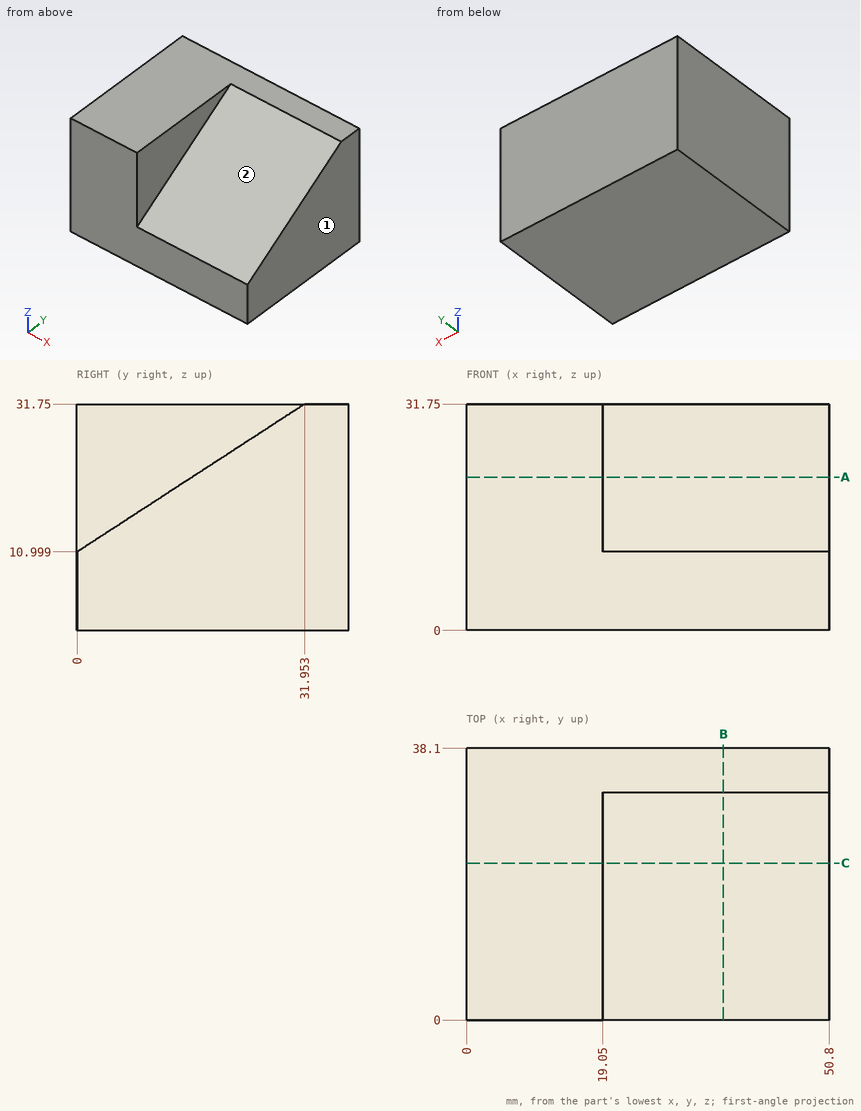
Here's the drawing with two shaded views (mm, measured from the low corner). I have some questions. A direction names the side the tool comes from. Give positions to 0.01 mm unless a question says otherwise; leave off trailing zeros. Loops run counter-clockwise (first coordinate to the right, second up) from the corner with the lowest first, then second, coordinate; pieces in that order, holes last. Notation, with made-up numbers: (64.25, -0.5) - (103.25, -0.5) arc R13 cw to (103.25, 8.5) - close; hole circle Ø2 at (-36, 86.25). An arc over 180 degrees is marked (long way). One line per item, written item: value.
(1) If we section it at B-B, the plane x = 36: List the corners of the cut face in (y, z) for me.
Verdict:
outline: (0, 0) - (38.1, 0) - (38.1, 31.75) - (31.95, 31.75) - (0, 11) - close
(2) I'm going to push flat-ended pins straight in: pin 1 (1 mm diameter, centred on y = 11, z = 6.5, fed in from -X); pin 2 (1 mm diameter, centred on y = 4, z = 27, fed in from +X); pin 3 (1 mm diameter, centred on x = 37.5, z = 23.5, fed in from -Y). Where does each tip first touch, or does it pass through?
Verdict:
pin 1: x = 0
pin 2: x = 19.05
pin 3: y = 18.48
(3) On a 3-axis mill with a long thin cutter (end or side, diameter ignored), from which of +Z, -Z, +X, -X, +Y, -Y can I reach the whole of each face in a straight line? I mean the marked faces 1 and 2. Say none if no direction works.
Verdict:
face 1: +Z, -Z, +X, +Y, -Y
face 2: +Z, +X, -Y
(4) If we section it at A-A, the plane z = 21.5: List the corners of the cut face in (x, y) for me, plus the area to 3 significant figures.
Verdict:
outline: (0, 0) - (19.05, 0) - (19.05, 16.17) - (50.8, 16.17) - (50.8, 38.1) - (0, 38.1) - close
area: 1,420 mm^2
(5) If we section it at C-C, the plane y = 22: List the corners of the cut face in (x, z) for me.
Verdict:
outline: (0, 0) - (50.8, 0) - (50.8, 25.29) - (19.05, 25.29) - (19.05, 31.75) - (0, 31.75) - close
(6) I need wall thicknesses on line 1 along X through (y, z) = (6, 29.5); line 2 along Z through (x, y) = (44, 23); line 3 along Z through (x, y) = (47, 9.5). Which ranges of each line are inside material? Lowest first, please.
Verdict:
line 1: 0 to 19.05
line 2: 0 to 25.94
line 3: 0 to 17.17
